Source: CAD feature listing. Evaluate the final solid. Frame: model axes, mm. A direction names the side the tool comes from. Give positions to 0.01 mm unless a question says otherwise; leave off trailing zeros. Write each loop counter-clockwise with the first axis right and the second up, starting at its lowest first coordinate (ties: lowest second). Pieces come first, ordered by that corner, then holes. Notation, with made-up numbers: (7, 19) -> (32, 19) arc R20 ccw to (32, 51) -> close; hole circle Ø5 at (42, 51.5). An arc over 180 degrees is marked (long way). Answer as a JSON object with one key per item and string values. Group by question number.
Item 1: Access query for faces 1 (the face through (1.3, -1.3, 15)), 2 (the face through (-1.19, -5.37, 24.61)), 3 (the face through (-0.13, -11.24, 3.49)). Directions: +Z, -Z, +X, -X, +Y, -Y. A direction counts if a zero-diameter tool reaches every point of the face in a straight line with its end or side. Return the directions, or none.
Item 2: First-contact query: pin 1 Ø3 at (y, z) = (6, 21) entering from +X; pin 2 Ø2 at (x, y) = (-4, 6) entering from -Z; pin 3 Ø3 at (y, z) = (0, 2.5) entering from +X; pin 4 Ø6 at (y, z) = (-5.5, 13.5) entering from +X. Flat tips, straight axial feed; report the tip coordinate or a pass-through.
Item 3: Section query C-C on z = 29.5. Return the cut outline in (x, y).
Item 4: Ray query, probe 1 along Y at (x, z) = (0, 1.45); probe 2 along Y at (x, z) = (0, 31.25); probe 3 along Z at (x, y) = (10.75, 0.75). Return the intervals inside material, ascending. Write a range as from..to.
Item 5: Section query A-A on x = 0. Return the cut outline in (y, z), plus the area to 3 significant figures.
Item 6: Section query D-D on z = 8. Return the cut outline in (x, y), plus the area to 3 significant figures.
Item 7: Section query B-B on z = 2.5. Return the cut outline in (x, y), plus the area to 3 significant figures.
Item 8: Pull-direction query (Y, two-part tool) for faces 4 (the face through (-1.2, 1.2, 35)), 5 (the face through (-3.27, -2.51, 13.4)), 6 (the face through (-1.266, -5.701, 14.514)); classes: pulls with the +Y half, pulls with the -Y half, needs draft (parallel to the pull), parting line crosses it, or undercut.
from build123d import *

# Parameters (mm, degrees)
F0_R      = 12.5
F0_R_2    = 10
F1_DEPTH  = 5
F4_R      = 12.5
F3_R      = 5.5
F6_R      = 10
F7_R      = 3
F9_R      = 5.5
F10_DEPTH = 20
F11_SIZE  = 0.5
F12_R     = 1
F13_DEPTH = 25
F14_R     = 1
F15_DEPTH = 25
F16_R     = 1.5
F17_DEPTH = 35.001


with BuildPart() as f1:
    # F0 (on Top) → F1 (new body)
    with BuildSketch(Plane.XY):
        Circle(F0_R)
        Circle(F0_R_2, mode=Mode.SUBTRACT)
    extrude(amount=F1_DEPTH)

    # F4 (on face) → F5 section 0
    with BuildSketch(Plane.XY.offset(5)):
        Circle(F4_R)
    # F3 (on offset) → F5 section 1
    with BuildSketch(Plane.XY.offset(15)):
        Circle(F3_R)
    loft()

    # F6 (on face) → F8 section 0
    with BuildSketch(Plane.XY.offset(5)):
        Circle(F6_R)
    # F7 (on offset) → F8 section 1
    with BuildSketch(Plane.XY.offset(15)):
        Circle(F7_R)
    loft(mode=Mode.SUBTRACT)

    # F9 (on face) → F10 (join)
    with BuildSketch(Plane.XY.offset(15)):
        Circle(F9_R)
    extrude(amount=F10_DEPTH)

    # F11
    f11_edges = [f1.edges().sort_by_distance(p)[0] for p in [
        (-5.5, 0, 35),
    ]]
    chamfer(f11_edges, length=F11_SIZE)

    # F12 (on Right) → F13 (cut, symmetric)
    with BuildSketch(Plane.YZ):
        with Locations((0, 2.5)):
            Circle(F12_R)
    extrude(amount=F13_DEPTH, both=True, mode=Mode.SUBTRACT)

    # F14 (on Front) → F15 (cut, symmetric)
    with BuildSketch(Plane.XZ):
        with Locations((0, 2.5)):
            Circle(F14_R)
    extrude(amount=F15_DEPTH, both=True, mode=Mode.SUBTRACT)

    # F16 (on face) → F17 (cut, through all)
    with BuildSketch(Plane.XY.offset(35)):
        Circle(F16_R)
    extrude(amount=-F17_DEPTH, mode=Mode.SUBTRACT)


solid = f1.part
Worked answers:
{
 "1": {"face 1": "-Z", "face 2": "+Z", "face 3": "+Y, -Y"},
 "2": {"pin 1": "x = 3.16", "pin 2": "z = 7.56", "pin 3": "x = 12.5", "pin 4": "x = 7.36"},
 "3": {"outline": "circle Ø11 at (0, 0); hole circle Ø3 at (0, 0)"},
 "4": {"probe 1": "-12.5..-10, 10..12.5", "probe 2": "-5.5..-1.5, 1.5..5.5", "probe 3": "0..1.84, 3.16..7.46"},
 "5": {"outline": "(-12.5, 0) -> (-10, 0) -> (-10, 1.5) -> (-12.5, 1.5) -> close; (-12.5, 3.5) -> (-10, 3.5) -> (-10, 5) -> (-3, 15) -> (-1.5, 15) -> (-1.5, 35) -> (-5, 35) -> (-5.5, 34.5) -> (-5.5, 15) -> (-12.5, 5) -> close; (1.5, 15) -> (3, 15) -> (10, 5) -> (10, 3.5) -> (12.5, 3.5) -> (12.5, 5) -> (5.5, 15) -> (5.5, 34.5) -> (5, 35) -> (1.5, 35) -> close; (10, 0) -> (12.5, 0) -> (12.5, 1.5) -> (10, 1.5) -> close", "area": "225 mm^2"},
 "6": {"outline": "circle Ø20.8 at (0, 0); hole circle Ø15.8 at (0, 0)", "area": "144 mm^2"},
 "7": {"outline": "(-12.46, -1) arc R12.5 ccw to (-1, -12.46) -> (-1, -9.95) arc R10 cw to (-9.95, -1) -> close; (-12.46, 1) -> (-9.95, 1) arc R10 cw to (-1, 9.95) -> (-1, 12.46) arc R12.5 ccw to start; (1, -12.46) arc R12.5 ccw to (12.46, -1) -> (9.95, -1) arc R10 cw to (1, -9.95) -> close; (1, 9.95) arc R10 cw to (9.95, 1) -> (12.46, 1) arc R12.5 ccw to (1, 12.46) -> close", "area": "157 mm^2"},
 "8": {"face 4": "needs draft", "face 5": "undercut", "face 6": "parting line crosses it"}
}
